from build123d import *

# Parameters (mm, degrees)
F0_W     = 165.6668949872
F0_H     = 9.4798584469
F1_DEPTH = 25.4
F2_R     = 5.1477874533
F3_DEPTH = 25.4
F4_R     = 5.221731546
F5_DEPTH = 25.4


with BuildPart() as f1:
    # F0 (on Front) → F1 (new body)
    with BuildSketch(Plane.XZ):
        with Locations((52.3083051667, 9.6694554668)):
            Rectangle(F0_W, F0_H)
    extrude(amount=F1_DEPTH)

    # F2 (on face) → F3 (cut)
    with BuildSketch(Plane(origin=(0, 0, 4.9295262434), x_dir=(1, 0, 0), z_dir=(0, 0, -1))):
        with Locations((-24.3377815932, 12.8386663273)):
            Circle(F2_R)
    extrude(amount=-F3_DEPTH, mode=Mode.SUBTRACT)

    # F4 (on face) → F5 (cut)
    with BuildSketch(Plane.XY.offset(14.4093846902)):
        with Locations((128.8211345673, -13.5866040364)):
            Circle(F4_R)
    extrude(amount=-F5_DEPTH, mode=Mode.SUBTRACT)


solid = f1.part
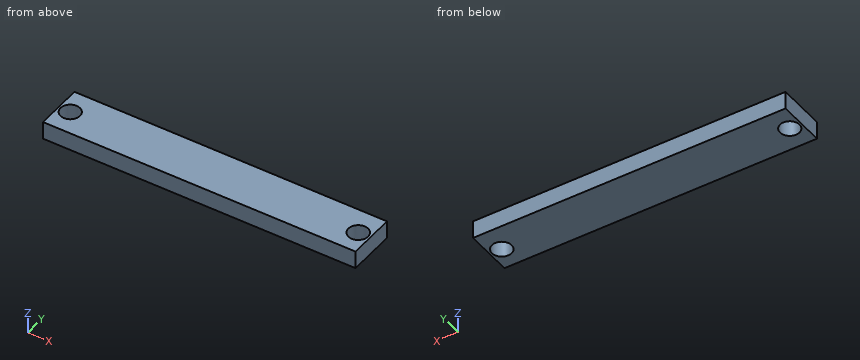
Work out the finished part from the listing and answer in its coordinate system (mm). Give positions to 0.01 mm unless a question says otherwise; leave off trailing zeros. Order: outer loops, then holes, each group sorted by start corner. A loop starts at its lowest first (then second) coordinate and runs counter-clockwise, first axis right, second up. Notation, with made-up numbers: M 76.5,17 L 135.5,17 A16 cw 135.5,34 Z; hole C 55,-28 d3. An arc over 180 degrees is marked long. Return JSON: item names as keys, results as strings.
Q1. Find section A-A, the plane y = -11.25. Write down the section's boundary in (x, z).
Answer below:
{"outline": "M -30.53,4.93 L -29.23,4.93 L -29.23,14.41 L -30.53,14.41 Z; M -19.44,4.93 L 124.15,4.93 L 124.15,14.41 L -19.44,14.41 Z; M 133.49,4.93 L 135.14,4.93 L 135.14,14.41 L 133.49,14.41 Z"}
Q2. Find the intervals of material crossed by line 1 along X through (y, z) = (-14.75, 9.75); line 2 along X through (y, z) = (-17, 6.75), in increasing order. Write a range as [from, to].
Answer below:
{"line 1": "x = [-30.53, -29.12], [-19.56, 123.73], [133.91, 135.14]", "line 2": "x = [-30.53, -27.37], [-21.31, 124.87], [132.77, 135.14]"}
Q3. Each of these flat-tipped pins is pushed along its axis until it touches: pin 1 (9.5 mm diameter, centred on x = -24.34, y = -12.84, fed in from +Z); pin 2 (2 mm diameter, centred on x = 68, z = 8, fed in from +Y). Where does it stop, or does it pass through?
Answer below:
{"pin 1": "passes through", "pin 2": "stops at y = 0"}
Q4. Find section B-B, the plane z = 9.25. Write down the section's boundary in (x, y).
Answer below:
{"outline": "M -30.53,-25.4 L 135.14,-25.4 L 135.14,0 L -30.53,0 Z; hole C -24.34,-12.84 d10.3; hole C 128.82,-13.59 d10.44"}
